```python
from build123d import *

# Parameters (mm, degrees)
SKETCH1_R           = 15.24
BOSS_EXTRUDE1_DEPTH = 122.428
SKETCH2_W           = 50.8
SKETCH2_H           = 50.8
BOSS_EXTRUDE2_DEPTH = 3.175
SKETCH3_R           = 4
BOSS_EXTRUDE3_DEPTH = 21.336
CUT_EXTRUDE1_DEPTH  = 21.336
CUT_EXTRUDE2_DEPTH  = 3.175


with BuildPart() as part:
    # Sketch1 → Boss-Extrude1 (new body)
    with BuildSketch(Plane(origin=(0, 0, 0), x_dir=(1, 0, 0), z_dir=(0, 1, 0))):
        Circle(SKETCH1_R)
    extrude(amount=BOSS_EXTRUDE1_DEPTH)

    # Sketch2 → Boss-Extrude2 (add)
    with BuildSketch(Plane(origin=(0, 122.428, 0), x_dir=(1, 0, 0), z_dir=(0, 1, 0))):
        Rectangle(SKETCH2_W, SKETCH2_H)
    extrude(amount=BOSS_EXTRUDE2_DEPTH)

    # Sketch3 → Boss-Extrude3 (add)
    with BuildSketch(Plane(origin=(0, 125.603, 0), x_dir=(1, 0, 0), z_dir=(0, 1, 0))):
        Circle(SKETCH3_R)
    extrude(amount=BOSS_EXTRUDE3_DEPTH)

    # Sketch4 → Cut-Extrude1 (cut)
    with BuildSketch(Plane(origin=(0, 146.939, 0), x_dir=(1, 0, 0), z_dir=(0, 1, 0))):
        with BuildLine():
            Line((2.645751311, 3), (-2.645751311, 3))
            ThreePointArc((-2.645751311, 3), (0, 4), (2.645751311, 3))
        make_face()
    extrude(amount=-CUT_EXTRUDE1_DEPTH, mode=Mode.SUBTRACT)

    # Sketch5 → Cut-Extrude2 (cut)
    with BuildSketch(Plane(origin=(0, 125.603, 0), x_dir=(1, 0, 0), z_dir=(0, 1, 0))):
        with BuildLine():
            Line((-16.764, 18.288), (-16.764, 7.366))
            ThreePointArc((-16.764, 7.366), (-18.542, 5.588), (-20.32, 7.366))
            Line((-20.32, 7.366), (-20.32, 18.288))
            ThreePointArc((-20.32, 18.288), (-18.542, 20.066), (-16.764, 18.288))
        make_face()
        with BuildLine():
            Line((-16.764, -7.112), (-16.764, -18.034))
            ThreePointArc((-16.764, -18.034), (-18.542, -19.812), (-20.32, -18.034))
            Line((-20.32, -18.034), (-20.32, -7.112))
            ThreePointArc((-20.32, -7.112), (-18.542, -5.334), (-16.764, -7.112))
        make_face()
        with BuildLine():
            Line((19.812, -7.112), (19.812, -18.034))
            ThreePointArc((19.812, -18.034), (18.034, -19.812), (16.256, -18.034))
            Line((16.256, -18.034), (16.256, -7.112))
            ThreePointArc((16.256, -7.112), (18.034, -5.334), (19.812, -7.112))
        make_face()
        with BuildLine():
            Line((19.812, 18.288), (19.812, 7.366))
            ThreePointArc((19.812, 7.366), (18.034, 5.588), (16.256, 7.366))
            Line((16.256, 7.366), (16.256, 18.288))
            ThreePointArc((16.256, 18.288), (18.034, 20.066), (19.812, 18.288))
        make_face()
    extrude(amount=-CUT_EXTRUDE2_DEPTH, mode=Mode.SUBTRACT)


solid = part.part
```
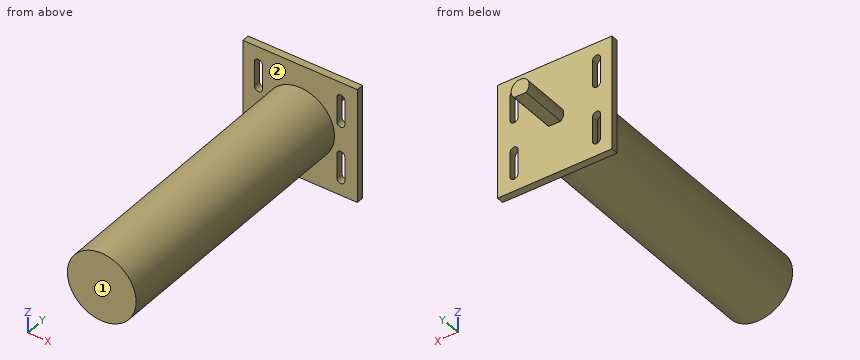
Check sheet for the modelled part. Datum: model origin and axes. Units: mm. Face numbers are marked on the shaded views. A direction names the side the tool comes from. Round coordinates to 2 decimals unless told otherwise and drop trailing zeros. Loops run counter-clockwise (first coordinate to the right, second up) from the corner with the lowest first, then second, coordinate; pieces in that order, holes last. Notation, with made-up numbers: (-24, 12.5) -> (16, 12.5) arc R20 ccw to (16, 30.5) -> close; hole circle Ø5 at (37.25, 33). An arc over 180 degrees is marked (long way). Write item = value, one per line. Start each with the question number.
1) Thickness scan on probe 1 along Z at (x, y) = (-18.5, 123.5); probe 2 along Y at (x, z) = (-9.5, 3.5); probe 3 along Y at (x, z) = (-22.5, 19). Record the ranges inside material, lowest first.
2) Set-up check for the marked faces 1 and 2: record each of +Z, -Z, +X, -X, +Y, -Y from which the full face is reachable in a straight line by a thin tool's end or side.
3) Sectioned sample at D-D, the plane y = 134. Record the cut outline in (x, z), plus the area to 3 significant figures.
4) Sectioned sample at B-B, the plane z = 0. Record the cut outline in (x, y).
5) Gauge pin test, flat ends, axial feed: pin 1 Ø5 at (y, z) = (84.5, 9.5) entering from -X; pin 2 Ø1.5 at (x, y) = (11, 119.5) entering from +Z; pin 3 Ø4 at (x, z) = (-14, -1.5) entering from -Y; pin 4 Ø4 at (x, y) = (-16, 81.5) entering from -Z. Record the tip position at first contact, or that the pin passes through.
6) Sectioned sample at A-A, the plane z = 11. Record the cut outline in (x, y).
7) Sectioned sample at C-C, the plane x = 0. Record the cut outline in (y, z), plus the area to 3 significant figures.
Results are:
q1.probe_1 = -25.4 to -20.07, -5.59 to 5.33, 19.81 to 25.4
q1.probe_2 = 0 to 125.6
q1.probe_3 = 122.43 to 125.6
q2.face_1 = +Z, -Z, +X, -X, -Y
q2.face_2 = -Y
q3.outline = (-2.65, -3) -> (2.65, -3) arc R4 ccw (long way) to start
q3.area = 46.6 mm^2
q4.outline = (-25.4, 122.43) -> (-15.24, 122.43) -> (-15.24, 0) -> (15.24, 0) -> (15.24, 122.43) -> (25.4, 122.43) -> (25.4, 125.6) -> (4, 125.6) -> (4, 146.94) -> (-4, 146.94) -> (-4, 125.6) -> (-25.4, 125.6) -> close
q5.pin_1 = -13.54
q5.pin_2 = 11.28
q5.pin_3 = 0
q5.pin_4 = -6.02
q6.outline = (-25.4, 122.43) -> (-20.32, 122.43) -> (-20.32, 125.6) -> (-25.4, 125.6) -> close; (-16.76, 122.43) -> (-10.55, 122.43) -> (-10.55, 0) -> (10.55, 0) -> (10.55, 122.43) -> (16.26, 122.43) -> (16.26, 125.6) -> (-16.76, 125.6) -> close; (19.81, 122.43) -> (25.4, 122.43) -> (25.4, 125.6) -> (19.81, 125.6) -> close
q7.outline = (0, -15.24) -> (122.43, -15.24) -> (122.43, -25.4) -> (125.6, -25.4) -> (125.6, -3) -> (146.94, -3) -> (146.94, 4) -> (125.6, 4) -> (125.6, 25.4) -> (122.43, 25.4) -> (122.43, 15.24) -> (0, 15.24) -> close
q7.area = 4,040 mm^2
